The model under review builds one solid part; all positions refer to its coordinate system, in mm. Give positions to 0.01 mm unless a question says otherwise; leave off trailing zeros. Put each result on its own line as item: value.
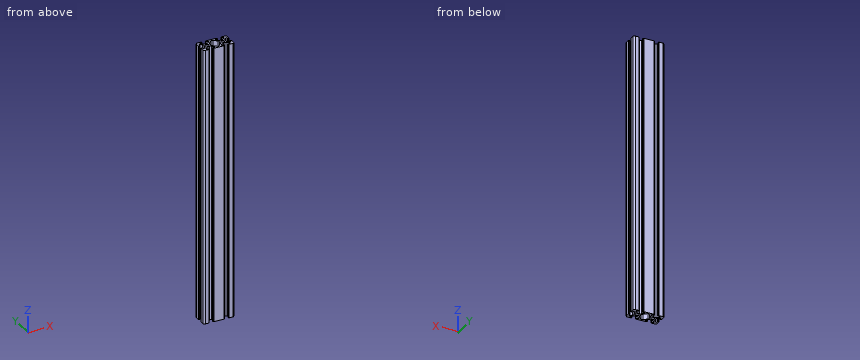
```python
from build123d import *

# Parameters (mm, degrees)
CROQUIS1_R              = 2.15
SALIENTE_EXTRUIR1_DEPTH = 360


with BuildPart() as part:
    # Croquis1 → Saliente-Extruir1 (new body)
    with BuildSketch(Plane.XY.offset(20)):
        with BuildLine():
            Line((32.499999987, 1.499999997), (32.499999987, 0.800000002))
            ThreePointArc((32.499999987, 0.800000002), (32.734314563, 0.234314576), (33.29999999, 0))
            Line((33.29999999, 0), (38, 0))
            ThreePointArc((38, 0), (39.414213562, 0.585786438), (40, 2))
            Line((40, 2), (40, 6.700000003))
            ThreePointArc((40, 6.700000003), (39.765685425, 7.265685427), (39.2, 7.500000003))
            Line((39.2, 7.500000003), (38.499999996, 7.500000003))
            ThreePointArc((38.499999996, 7.500000003), (38.287867962, 7.412132037), (38.199999996, 7.200000003))
            Line((38.199999996, 7.200000003), (38.199999996, 5.082411612))
            ThreePointArc((38.199999996, 5.082411612), (37.686138518, 4.313363563), (36.778984492, 4.493807718))
            Line((36.778984492, 4.493807718), (34.528679652, 6.744112558))
            ThreePointArc((34.528679652, 6.744112558), (33.878361399, 7.717382603), (33.649999997, 8.865432898))
            Line((33.649999997, 8.865432898), (33.649999997, 11.134567109))
            ThreePointArc((33.649999997, 11.134567109), (33.878361399, 12.282617405), (34.528679653, 13.255887451))
            Line((34.528679653, 13.255887451), (36.778984498, 15.506192296))
            ThreePointArc((36.778984498, 15.506192296), (37.68613852, 15.686636451), (38.199999996, 14.917588405))
            Line((38.199999996, 14.917588405), (38.199999996, 12.800000003))
            ThreePointArc((38.199999996, 12.800000003), (38.287867963, 12.587867967), (38.499999999, 12.5))
            Line((38.499999999, 12.5), (39.199999998, 12.5))
            ThreePointArc((39.199999998, 12.5), (39.765685424, 12.734314576), (40, 13.300000002))
            Line((40, 13.300000002), (40, 18))
            ThreePointArc((40, 18), (39.414213562, 19.414213562), (38, 20))
            Line((38, 20), (33.299999987, 20))
            ThreePointArc((33.299999987, 20), (32.734314562, 19.765685425), (32.499999987, 19.2))
            Line((32.499999987, 19.2), (32.499999987, 18.499999997))
            ThreePointArc((32.499999987, 18.499999997), (32.587867953, 18.287867963), (32.799999987, 18.199999997))
            Line((32.799999987, 18.199999997), (34.917587986, 18.199999997))
            ThreePointArc((34.917587986, 18.199999997), (35.686635927, 17.686138592), (35.506191797, 16.778984693))
            Line((35.506191797, 16.778984693), (33.255886766, 14.528679662))
            ThreePointArc((33.255886766, 14.528679662), (32.282616721, 13.878361409), (31.134566426, 13.650000007))
            Line((31.134566426, 13.650000007), (28.86543289, 13.650000007))
            ThreePointArc((28.86543289, 13.650000007), (27.717382593, 13.878361409), (26.744112547, 14.528679663))
            Line((26.744112547, 14.528679663), (24.493807707, 16.778984503))
            ThreePointArc((24.493807707, 16.778984503), (24.313363553, 17.686138523), (25.082411597, 18.199999997))
            Line((25.082411597, 18.199999997), (27.199999997, 18.199999997))
            ThreePointArc((27.199999997, 18.199999997), (27.412132033, 18.287867964), (27.5, 18.5))
            Line((27.5, 18.5), (27.5, 19.199999998))
            ThreePointArc((27.5, 19.199999998), (27.265685424, 19.765685424), (26.699999997, 20))
            Line((26.699999997, 20), (13.299999987, 20))
            ThreePointArc((13.299999987, 20), (12.734314562, 19.765685425), (12.499999987, 19.2))
            Line((12.499999987, 19.2), (12.499999987, 18.499999997))
            ThreePointArc((12.499999987, 18.499999997), (12.587867953, 18.287867963), (12.799999987, 18.199999997))
            Line((12.799999987, 18.199999997), (14.917588389, 18.199999997))
            ThreePointArc((14.917588389, 18.199999997), (15.686636438, 17.686138519), (15.506192283, 16.778984493))
            Line((15.506192283, 16.778984493), (13.255887452, 14.528679662))
            ThreePointArc((13.255887452, 14.528679662), (12.282617407, 13.878361409), (11.134567112, 13.650000007))
            Line((11.134567112, 13.650000007), (8.86543289, 13.650000007))
            ThreePointArc((8.86543289, 13.650000007), (7.717382593, 13.878361409), (6.744112547, 14.528679663))
            Line((6.744112547, 14.528679663), (4.493807707, 16.778984503))
            ThreePointArc((4.493807707, 16.778984503), (4.313363553, 17.686138523), (5.082411597, 18.199999997))
            Line((5.082411597, 18.199999997), (7.199999997, 18.199999997))
            ThreePointArc((7.199999997, 18.199999997), (7.412132033, 18.287867964), (7.5, 18.5))
            Line((7.5, 18.5), (7.5, 19.199999998))
            ThreePointArc((7.5, 19.199999998), (7.265685424, 19.765685424), (6.699999997, 20))
            Line((6.699999997, 20), (2, 20))
            ThreePointArc((2, 20), (0.585786438, 19.414213562), (0, 18))
            Line((0, 18), (0, 13.3))
            ThreePointArc((0, 13.3), (0.234314575, 12.734314575), (0.8, 12.5))
            Line((0.8, 12.5), (1.500000005, 12.5))
            ThreePointArc((1.500000005, 12.5), (1.71213204, 12.587867966), (1.800000005, 12.8))
            Line((1.800000005, 12.8), (1.800000005, 14.91758839))
            ThreePointArc((1.800000005, 14.91758839), (2.313861483, 15.686636439), (3.22101551, 15.506192284))
            Line((3.22101551, 15.506192284), (5.471320341, 13.255887453))
            ThreePointArc((5.471320341, 13.255887453), (6.121638594, 12.282617408), (6.349999996, 11.134567113))
            Line((6.349999996, 11.134567113), (6.349999996, 8.865432892))
            ThreePointArc((6.349999996, 8.865432892), (6.121638593, 7.717382596), (5.47132034, 6.74411255))
            Line((5.47132034, 6.74411255), (3.2210155, 4.49380771))
            ThreePointArc((3.2210155, 4.49380771), (2.31386148, 4.313363556), (1.800000005, 5.0824116))
            Line((1.800000005, 5.0824116), (1.800000005, 7.2))
            ThreePointArc((1.800000005, 7.2), (1.712132039, 7.412132036), (1.500000003, 7.500000003))
            Line((1.500000003, 7.500000003), (0.800000003, 7.500000003))
            ThreePointArc((0.800000003, 7.500000003), (0.234314576, 7.265685427), (0, 6.7))
            Line((0, 6.7), (0, 2))
            ThreePointArc((0, 2), (0.585786438, 0.585786438), (2, 0))
            Line((2, 0), (6.7, 0))
            ThreePointArc((6.7, 0), (7.265685425, 0.234314575), (7.5, 0.8))
            Line((7.5, 0.8), (7.5, 1.5))
            ThreePointArc((7.5, 1.5), (7.412132034, 1.712132034), (7.2, 1.8))
            Line((7.2, 1.8), (5.0824116, 1.8))
            ThreePointArc((5.0824116, 1.8), (4.313363551, 2.313861478), (4.493807706, 3.221015504))
            Line((4.493807706, 3.221015504), (6.744112546, 5.471320344))
            ThreePointArc((6.744112546, 5.471320344), (7.717382591, 6.121638597), (8.865432886, 6.349999999))
            Line((8.865432886, 6.349999999), (11.134567108, 6.349999999))
            ThreePointArc((11.134567108, 6.349999999), (12.282617404, 6.121638597), (13.25588745, 5.471320343))
            Line((13.25588745, 5.471320343), (15.506192295, 3.221015498))
            ThreePointArc((15.506192295, 3.221015498), (15.686636449, 2.313861476), (14.917588403, 1.8))
            Line((14.917588403, 1.8), (12.79999999, 1.8))
            ThreePointArc((12.79999999, 1.8), (12.587867954, 1.712132033), (12.499999987, 1.499999997))
            Line((12.499999987, 1.499999997), (12.499999987, 0.800000003))
            ThreePointArc((12.499999987, 0.800000003), (12.734314563, 0.234314576), (13.29999999, 0))
            Line((13.29999999, 0), (26.7, 0))
            ThreePointArc((26.7, 0), (27.265685425, 0.234314575), (27.5, 0.8))
            Line((27.5, 0.8), (27.5, 1.5))
            ThreePointArc((27.5, 1.5), (27.412132034, 1.712132034), (27.2, 1.8))
            Line((27.2, 1.8), (25.0824116, 1.8))
            ThreePointArc((25.0824116, 1.8), (24.313363551, 2.313861478), (24.493807706, 3.221015504))
            Line((24.493807706, 3.221015504), (26.744112546, 5.471320344))
            ThreePointArc((26.744112546, 5.471320344), (27.717382591, 6.121638597), (28.865432886, 6.349999999))
            Line((28.865432886, 6.349999999), (31.134567114, 6.349999999))
            ThreePointArc((31.134567114, 6.349999999), (32.282617411, 6.121638597), (33.255887457, 5.471320343))
            Line((33.255887457, 5.471320343), (35.506192392, 3.221015408))
            ThreePointArc((35.506192392, 3.221015408), (35.686636535, 2.313861443), (34.917588538, 1.8))
            Line((34.917588538, 1.8), (32.79999999, 1.8))
            ThreePointArc((32.79999999, 1.8), (32.587867954, 1.712132033), (32.499999987, 1.499999997))
        make_face()
        with Locations((10, 10)):
            Circle(CROQUIS1_R, mode=Mode.SUBTRACT)
        with Locations((30, 10)):
            Circle(CROQUIS1_R, mode=Mode.SUBTRACT)
        with BuildLine():
            Line((18.585786097, 2.687006113), (14.528679097, 6.744113113))
            ThreePointArc((14.528679097, 6.744113113), (13.878360843, 7.717383159), (13.649999441, 8.865433456))
            Line((13.649999441, 8.865433456), (13.649999441, 11.134566554))
            ThreePointArc((13.649999441, 11.134566554), (13.878360843, 12.282616849), (14.528679096, 13.255886895))
            Line((14.528679096, 13.255886895), (18.585786441, 17.312994239))
            ThreePointArc((18.585786441, 17.312994239), (20.000000001, 17.898780676), (21.414213561, 17.312994239))
            Line((21.414213561, 17.312994239), (25.471320216, 13.255887584))
            ThreePointArc((25.471320216, 13.255887584), (26.12163847, 12.282617538), (26.349999872, 11.13456724))
            Line((26.349999872, 11.13456724), (26.349999872, 8.865433454))
            ThreePointArc((26.349999872, 8.865433454), (26.12163847, 7.717383158), (25.471320217, 6.744113113))
            Line((25.471320217, 6.744113113), (21.414213217, 2.687006113))
            ThreePointArc((21.414213217, 2.687006113), (19.999999657, 2.101219676), (18.585786097, 2.687006113))
        make_face(mode=Mode.SUBTRACT)
    extrude(amount=-SALIENTE_EXTRUIR1_DEPTH)


solid = part.part
```
(1) Wall thickness on L1, parallel to Y at x = 17, z = 5; L2, parallel to Y at x = 13, z = -187.5; L3, parallel to Y at x = 10, z = -91.5: over which ranges is each line inside the solid? List them lowest first.
The answers:
L1: 0 to 4.27, 15.73 to 20
L2: 0.06 to 1.8, 5.7 to 14.3, 18.2 to 19.94
L3: 6.35 to 7.85, 12.15 to 13.65
(2) Clearance check with flat-ended pins moving along their axes: pin 1 Ø0.6 at (x, z) = (1, -174) entering from -Y; pin 2 Ø0.6 at (y, z) = (1, -170) entering from +X; pin 3 Ø0.7 at (y, z) = (10, -179) entering from -X. State where each tip first meets the part, or that it passes through.
The answers:
pin 1: y = 0.13
pin 2: x = 39.87
pin 3: x = 6.35
(3) Take a section at A-A, the plane z = -214.5. Count the separate pieces of the cut face and the enclosed holes in it, then the cut area to 3 significant figures.
The answers:
separate pieces: 1
enclosed holes: 3
area: 332 mm^2
